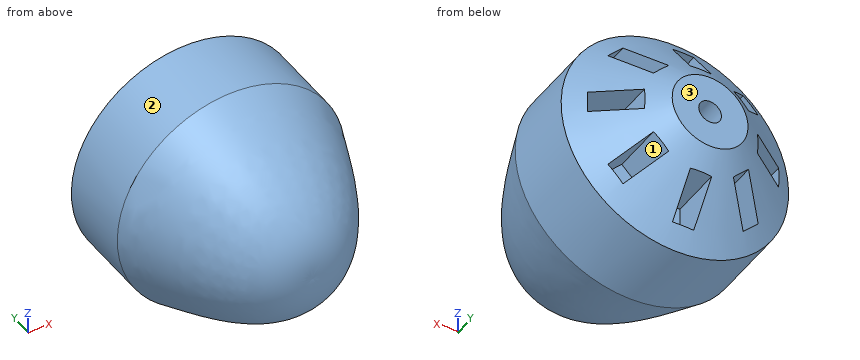
```python
from build123d import *

# Parameters (mm, degrees)
CUT_EXTRUDE_1_DEPTH      = 10
CUT_EXTRUDE_1_DEPTH_BACK = 1
SKETCH_3_R               = 1.5
CUT_EXTRUDE_START        = -1
SKETCH_4_W               = 2.811133726
SKETCH_4_H               = 5.156078578
CUT_EXTRUDE_2_DEPTH      = 36.217034404
PATTERN_CIRCULAR_1_COUNT = 8


with BuildPart() as part:
    # 草图1 → 旋转3 (revolve)
    with BuildSketch(Plane.XY, mode=Mode.PRIVATE) as revolve_3_sk:
        with BuildLine():
            Line((-15, 0.182551999), (-5, 7.680235811))
            Line((-5, 7.680235811), (0, 7.680235811))
            Line((0, 7.680235811), (0, -9.593702865))
            Line((0, -9.593702865), (0, -26.791420925))
            add(Edge.make_bspline(
                [(0, -26.791420925), (-8.890332256, -27.786972395), (-12.567592708, -15.34792859), (-15, -9.593702865)],
                knots=[0, 0, 0, 0, 1, 1, 1, 1], degree=3))
            Line((-15, -9.593702865), (-15, -6.069622936))
            Line((-15, -6.069622936), (-15, -3.569622936))
            Line((-15, -3.569622936), (-15, 0.182551999))
        make_face()
    revolve(revolve_3_sk.sketch.rotate(Axis((0, -9.593702865, 0), (0, 1, 0)), 270), axis=Axis((0, -9.593702865, 0), (0, 1, 0)))

    # 草图3 → 切除-拉伸1 (cut, two sides: drawn at the far end of the back side and taken through both)
    with BuildSketch(Plane(origin=(0, 0, 0), x_dir=(1, 0, 0), z_dir=(0, 1, 0)).offset(-CUT_EXTRUDE_1_DEPTH_BACK)):
        with Locations(Location((0, 0, 0), (0, 0, 90))):
            Circle(SKETCH_3_R)
    extrude(amount=CUT_EXTRUDE_1_DEPTH + CUT_EXTRUDE_1_DEPTH_BACK, mode=Mode.SUBTRACT)

    # 草图4 → 切除-拉伸2 (cut)
    with BuildSketch(Plane(origin=(0, 0, 0), x_dir=(1, 0, 0), z_dir=(0, 1, 0)).offset(CUT_EXTRUDE_START)):
        with Locations((0, 10.028828945)):
            Rectangle(SKETCH_4_W, SKETCH_4_H)
    cut_extrude_2 = extrude(amount=CUT_EXTRUDE_2_DEPTH, mode=Mode.SUBTRACT)

    # 阵列(圆周)1: 切除-拉伸2 ×8 about axis
    pattern_circular_1_axis = Axis((0, 0, 0), (0, 1, 0))
    for i in range(1, PATTERN_CIRCULAR_1_COUNT):
        add(cut_extrude_2.rotate(pattern_circular_1_axis, i * 360 / PATTERN_CIRCULAR_1_COUNT), mode=Mode.SUBTRACT)


solid = part.part
```
Design review of the part built by this model. Coordinates are the model's own, in mm. Face numbers are marked on the shaded views. Coordinates: 2 decimals unless noted, no trailing zeros. Loops run counter-clockwise (first coordinate to the right, second up) from the corner with the lowest first, then second, coordinate; pieces in that order, holes last. Notation, with made-up numbers: (71, 24.5) -> (122, 24.5) arc R31 cw to (122, 54.5) -> close; hole circle Ø5 at (-40, 50). An arc over 180 degrees is marked (long way). Answer as a JSON object with one key per item and string values.
Q1. Clearance check with flat-ended pins moving along their axes: pin 1 Ø1.5 at (x, y) = (12, -4.5) entering from +Z; pin 2 Ø8 at (y, z) = (-10.5, 6) entering from -X; pin 3 Ø8 at (x, z) = (1, 10) entering from +Y. State where each tip first meets the part, or that it passes through.
Answer block:
{"pin 1": "stops at z = 9.92", "pin 2": "stops at x = -14.85", "pin 3": "stops at y = 6.89"}
Q2. To check wall thickness, follow L1, parallel to X at y = 1, z = 0; L2, parallel to X at y = 2.25, z = 0; L3, parallel to X at y = 0.5, z = -7. State the ranges of each line that lie inside material, in increasing order.
Answer block:
{"L1": "x = -13.91 to -12.61, -7.45 to -1.5, 1.5 to 7.45, 12.61 to 13.91", "L2": "x = -7.45 to -1.5, 1.5 to 7.45", "L3": "x = -12.79 to -8.99, -5.01 to 5.01, 8.99 to 12.79"}
Q3. The part is to be moulded in two halves that separate along X. For the marked faces 1, 2 and 3, say which applies: +X half, -X half, draft (parallel to the pull), parting line (faces both ways), or undercut.
Answer block:
{"face 1": "undercut", "face 2": "parting line", "face 3": "draft"}
Q4. Take a section at A-A on y = -4. Give the boundary of the cut face in (x, z), plus the area to 3 significant figures.
Answer block:
{"outline": "circle Ø30 at (0, 0)", "area": "707 mm^2"}
